Input: part model. Units: mm. Frame: model coordinates. Coordinates: 2 decimals unless noted, no trailing zeros. Order: outer loops, then holes, each group sorted by start corner. A loop starts at its lowest first (then second) coordinate and runs counter-clockwise, first axis right, second up. Notation, with made-up numbers: (29.5, 78.5) -> (67.5, 78.5) arc R20 cw to (67.5, 95.5) -> close; hole circle Ø3 at (62.25, 71.25). An arc over 180 degrees is marked (long way). One line per item, written item: value. Start each with the question number.
from build123d import *

# Parameters (mm, degrees)
SKETCH1_W           = 35
SKETCH1_H           = 50
SKETCH1_W_2         = 32
SKETCH1_H_2         = 47
BOSS_EXTRUDE1_DEPTH = 460
BOSS_EXTRUDE2_DEPTH = 3
SKETCH3_R           = 19
CUT_EXTRUDE1_DEPTH  = 3
SKETCH5_R           = 21
SKETCH5_R_2         = 17.5
BOSS_EXTRUDE7_DEPTH = 35
SKETCH6_R           = 19
CUT_EXTRUDE2_DEPTH  = 9
SKETCH1_2_W         = 35
SKETCH1_2_H         = 50
SKETCH1_2_W_2       = 32
SKETCH1_2_H_2       = 47
BOSS_EXTRUDE8_DEPTH = 390


with BuildPart() as part:
    # Sketch1 → Boss-Extrude1 (new body)
    with BuildSketch(Plane.XY):
        Rectangle(SKETCH1_W, SKETCH1_H)
        Rectangle(SKETCH1_W_2, SKETCH1_H_2, mode=Mode.SUBTRACT)
    extrude(amount=BOSS_EXTRUDE1_DEPTH)

    # Sketch2 → Boss-Extrude2 (add)
    with BuildSketch(Plane.ZY.offset(17.5)):
        with BuildLine():
            Line((1, 0), (7.296110466, 25))
            Line((7.296110466, 25), (18.5, 69.487344987))
            ThreePointArc((18.5, 69.487344987), (35, 82.347129464), (51.5, 69.487344987))
            Line((51.5, 69.487344987), (62.703889534, 25))
            Line((62.703889534, 25), (69, 0))
            Line((69, 0), (1, 0))
        make_face()
    boss_extrude2 = extrude(amount=BOSS_EXTRUDE2_DEPTH)

    # Sketch3 → Cut-Extrude1 (cut)
    with BuildSketch(Plane.ZY.offset(20.5)):
        with Locations(Location((35, 44, 0), (0, 0, 270))):
            Circle(SKETCH3_R)
    cut_extrude1 = extrude(amount=-CUT_EXTRUDE1_DEPTH, mode=Mode.SUBTRACT)

    # Mirror1: Boss-Extrude2, Cut-Extrude1 across plane
    add(boss_extrude2.mirror(Plane(origin=(0, 0, 0), x_dir=(0, 0, 1), z_dir=(1, 0, 0))))
    add(cut_extrude1.mirror(Plane(origin=(0, 0, 0), x_dir=(0, 0, 1), z_dir=(1, 0, 0))), mode=Mode.SUBTRACT)

    # Sketch5 → Boss-Extrude7 (add)
    with BuildSketch(Plane(origin=(-17.5, 0, 0), x_dir=(0, 0, -1), z_dir=(1, 0, 0))):
        with Locations((-35, 44)):
            Circle(SKETCH5_R)
        with Locations(Location((-35, 44, 0), (0, 0, 270))):
            Circle(SKETCH5_R_2, mode=Mode.SUBTRACT)
    extrude(amount=BOSS_EXTRUDE7_DEPTH)

    # Sketch6 → Cut-Extrude2 (cut)
    with BuildSketch(Plane(origin=(17.5, 0, 0), x_dir=(0, 0, -1), z_dir=(1, 0, 0))):
        with Locations(Location((-35, 44, 0), (0, 0, 270))):
            Circle(SKETCH6_R)
    cut_extrude2 = extrude(amount=-CUT_EXTRUDE2_DEPTH, mode=Mode.SUBTRACT)

    # Mirror2: Cut-Extrude2 across plane
    add(cut_extrude2.mirror(Plane(origin=(0, 0, 0), x_dir=(0, 0, 1), z_dir=(1, 0, 0))), mode=Mode.SUBTRACT)

    # Sketch1<2> → Boss-Extrude8 (add)
    with BuildSketch(Plane.XY):
        Rectangle(SKETCH1_2_W, SKETCH1_2_H)
        Rectangle(SKETCH1_2_W_2, SKETCH1_2_H_2, mode=Mode.SUBTRACT)
    extrude(amount=-BOSS_EXTRUDE8_DEPTH)


solid = part.part
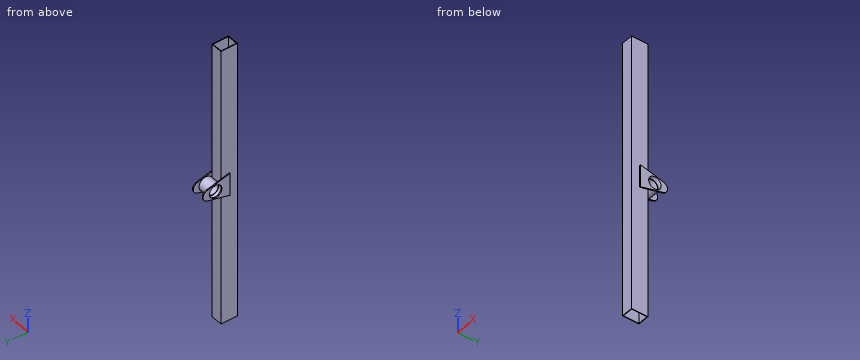
1) Section query A-A, the plane z = 100.5. Return the cut outline in (x, y), plus the area to 3 significant figures.
2) Pin query (flat end, axial travel): pin 1 Ø15 at (y, z) = (-1, 245) entering from -X; pin 2 Ø1 at (x, y) = (-3, 39) entering from +Z; pin 3 Ø3 at (y, z) = (-2, 293) entering from +X; pin 4 Ø2.5 at (x, z) = (18.5, 27.5) entering from -Y. Return the tip coordinate at first contact, or that it passes through.
3) Ray query, line 1 along Y through (x, z) = (-12.25, 35); line 2 along Y through (x, z) = (-3.5, 60); line 3 along Z through (x, y) = (15, 44). Return the intervals inside material, ascending. Write a range as from..to.
4) Section query B-B, the plane y = 44. Return the cut outline in (x, z).
Entries:
1. outline: (-17.5, -25) -> (17.5, -25) -> (17.5, 25) -> (-17.5, 25) -> close; hole (-16, -23.5) -> (16, -23.5) -> (16, 23.5) -> (-16, 23.5) -> close
1. area: 246 mm2
2. pin 1: stops at x = -17.5
2. pin 2: stops at z = 55.51
2. pin 3: stops at x = 17.5
2. pin 4: stops at y = -25
3. line 1: y = -25..-23.5, 23..25, 63..65
3. line 2: y = -25..-23.5, 23.5..25
3. line 3: z = 14..16, 54..56
4. outline: (-20.5, 12.08) -> (-17.5, 12.08) -> (-17.5, 14) -> (17.5, 14) -> (17.5, 12.08) -> (20.5, 12.08) -> (20.5, 16) -> (8.5, 16) -> (8.5, 17.5) -> (-8.5, 17.5) -> (-8.5, 16) -> (-20.5, 16) -> close; (-20.5, 54) -> (-8.5, 54) -> (-8.5, 52.5) -> (8.5, 52.5) -> (8.5, 54) -> (20.5, 54) -> (20.5, 57.92) -> (17.5, 57.92) -> (17.5, 56) -> (-17.5, 56) -> (-17.5, 57.92) -> (-20.5, 57.92) -> close
